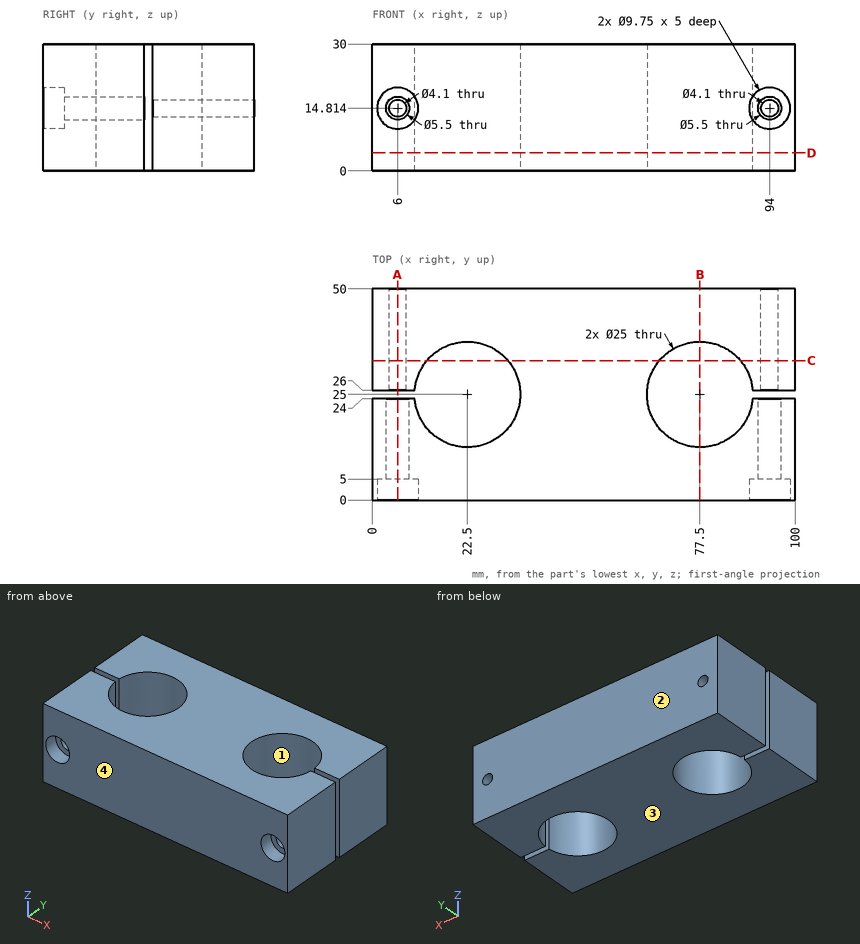
Source: three-view drawing plus pictorial views. Frame: mm from the lowest corner of the part. Give positions to 0.01 mm unless a question says otherwise; leave off trailing zeros. Order: outer loops, then holes, each group sorted by start corner. A loop starts at its lowest first (then second) coordinate and runs counter-clockwise, first axis right, second up. Notation, with made-up numbers: M 10,-8 L 54,-8 A26 cw 54,10 Z; hole C 22,53 d10. An arc over 180 degrees is marked long. Return JSON: item names as keys, results as strings.
Item 1: Ray query, probe 1 along Z at (x, y) = (94, 3.95); probe 2 along X at (y, z) = (22, 28) (1 decimal); probe 3 along Z at (x, y) = (6, 44) (1 decimal). Return the intervals inside material, ascending.
Solutions:
{"probe 1": "0 to 9.94, 19.69 to 30", "probe 2": "0 to 10.4, 34.6 to 65.4, 89.6 to 100", "probe 3": "0 to 12.8, 16.9 to 30"}
Item 2: Pull-direction query (Y, two-part tool) for the marked faces 1, 2, 3 and 4; classes: +Y half, -Y half, draft (parallel to the pull), parting line (faces both ways), or undercut.
Solutions:
{"face 1": "undercut", "face 2": "+Y half", "face 3": "draft", "face 4": "-Y half"}
Item 3: Cut plane B-B (x = 77.5). Return loops of the section in (y, z).
Solutions:
{"outline": "M 0,0 L 12.5,0 L 12.5,30 L 0,30 Z; M 37.5,0 L 50,0 L 50,30 L 37.5,30 Z"}
Item 4: Cut plane A-A (x = 6). Return loops of the section in (y, z) (1 decimal), then the cut area to 3 significant figures.
Solutions:
{"outline": "M 0,0 L 24,0 L 24,12.1 L 5,12.1 L 5,9.9 L 0,9.9 Z; M 0,19.7 L 5,19.7 L 5,17.6 L 24,17.6 L 24,30 L 0,30 Z; M 26,0 L 50,0 L 50,12.8 L 26,12.8 Z; M 26,16.9 L 50,16.9 L 50,30 L 26,30 Z", "area": "1,190 mm^2"}
Item 5: Cut plane D-D (z = 4.25). Return loops of the section in (x, y), then the cut area to 3 significant figures.
Solutions:
{"outline": "M 0,0 L 100,0 L 100,24 L 89.96,24 A12.5 cw long 89.96,26 L 100,26 L 100,50 L 0,50 L 0,26 L 10.04,26 A12.5 cw long 10.04,24 L 0,24 Z", "area": "3,980 mm^2"}
Item 6: First-contact query: P1, Ø3.5, axis at x = 6, z = 14.81, coming from the -Y side; P2, Ø9, axis at x = 94, z = 14.81, coming from the -Y side; P3, Ø4.5, axis at x = 94, z = 14.81, coming from the -Y side. Flat tips, straight axial feed; report the tip coordinate or a pass-through.
Solutions:
{"P1": "through", "P2": "y = 5", "P3": "y = 26"}
Item 7: Cut plane C-C (y = 33). State how many separate pieces and enclosed holes the cut face has, then the cut area to 3 significant figures.
Solutions:
{"separate pieces": "3", "enclosed holes": "2", "area": "1,820 mm^2"}
